Build history of the part. All positions in model axes, mm. Face numbers are marked on the shaded views. A direction names the side the tool comes from. Round coordinates to 2 decimals unless told otherwise and drop trailing zeros. Write each loop counter-clockwise with the first axis right and the second up, starting at its lowest first coordinate (ties: lowest second). Pieces come first, ordered by that corner, then holes.
1) Flat gauge pins, fed straight in: pin 1 (10 mm diameter, centred on y = 2, z = -17, fed in from +X); pin 2 (6 mm diameter, centred on x = 15, z = 27.5, fed in from -Y); pin 3 (7 mm diameter, centred on x = 0, z = 0, fed in from -Y); pin 4 (3 mm diameter, centred on x = 1.5, y = -0.5, fed in from -Z). Where does each tip first touch, or does it go through?
2) Wall check: probe 1 along Z at (x, y) = (0, 4); probe 2 along Z at (x, y) = (0, -4); probe 3 along Y at (x, z) = (10, 27.5). Give the ranges that are in metal, low to high.
3) Saw through at D-D (x = -28). Write the cut outline in (y, z).
4) Saw through at A-A (z = 1). Write the cut outline in (x, y).
5) Saw through at C-C (y = 12.5). Write the cut outline in (x, z).
6) Saw through at B-B (x = -1.5). Write the cut outline in (y, z), plus the area to 3 significant figures.
7) Which spindle directions (+Z, -Z, +X, -X, +Y, -Y) get a long thin tool onto all of the face, cutting with end or side? Do the marked faces 1 and 2. Say none if no direction does.
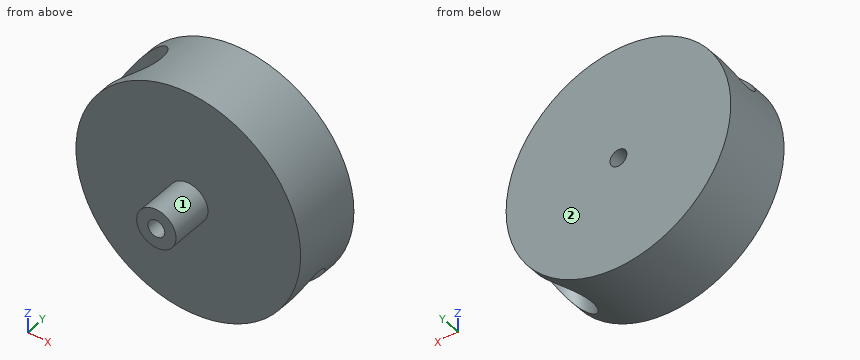
from build123d import *

# Parameters (mm, degrees)
SKETCH1_R           = 40
SKETCH1_R_2         = 3
BOSS_EXTRUDE1_DEPTH = 25
SKETCH2_R           = 7
SKETCH2_R_2         = 3
BOSS_EXTRUDE2_DEPTH = 15
SKETCH3_R           = 9
CUT_EXTRUDE1_DEPTH  = 41
SKETCH4_R           = 9
CUT_EXTRUDE2_DEPTH  = 41.0000001


with BuildPart() as part:
    # Sketch1 → Boss-Extrude1 (new body)
    with BuildSketch(Plane(origin=(0, 0, 0), x_dir=(1, 0, 0), z_dir=(0, 1, 0))):
        Circle(SKETCH1_R)
        Circle(SKETCH1_R_2, mode=Mode.SUBTRACT)
    extrude(amount=BOSS_EXTRUDE1_DEPTH)

    # Sketch2 → Boss-Extrude2 (add)
    with BuildSketch(Plane.XZ):
        Circle(SKETCH2_R)
        Circle(SKETCH2_R_2, mode=Mode.SUBTRACT)
    extrude(amount=BOSS_EXTRUDE2_DEPTH)

    # Sketch3 → Cut-Extrude1 (cut, through all)
    with BuildSketch(Plane.XY):
        with Locations((28, 12.5)):
            Circle(SKETCH3_R)
    extrude(amount=-CUT_EXTRUDE1_DEPTH, mode=Mode.SUBTRACT)

    # Sketch4 → Cut-Extrude2 (cut, through all)
    with BuildSketch(Plane.XY):
        with Locations((-28, 12.5)):
            Circle(SKETCH4_R)
    extrude(amount=CUT_EXTRUDE2_DEPTH, mode=Mode.SUBTRACT)


solid = part.part
Evaluation:
1. pin 1: stops at x = 38.16
1. pin 2: stops at y = 0
1. pin 3: stops at y = -15
1. pin 4: stops at z = -40
2. probe 1: z = -40 to -3, 3 to 40
2. probe 2: z = -7 to -3, 3 to 7
2. probe 3: y = 0 to 25
3. outline: (0, -28.57) - (25, -28.57) - (25, 28.57) - (21.5, 28.57) - (21.5, 0) - (3.5, 0) - (3.5, 28.57) - (0, 28.57) - close
4. outline: (-39.99, 0) - (-6.93, 0) - (-6.93, -15) - (-2.83, -15) - (-2.83, 25) - (-39.99, 25) - close; (2.83, -15) - (6.93, -15) - (6.93, 0) - (39.99, 0) - (39.99, 25) - (2.83, 25) - close; hole circle Ø18 at (-28, 12.5)
5. outline: (-37, 0) - (-37, 15.2) arc R40 ccw to (19, -35.2) - (19, 0) - (37, 0) - (37, -15.2) arc R40 ccw to (-19, 35.2) - (-19, 0) - close; hole circle Ø6 at (0, 0)
6. outline: (-15, -6.84) - (0, -6.84) - (0, -39.97) - (25, -39.97) - (25, -2.6) - (-15, -2.6) - close; (-15, 2.6) - (25, 2.6) - (25, 39.97) - (0, 39.97) - (0, 6.84) - (-15, 6.84) - close
6. area: 2,000 mm2
7. face 1: -Y
7. face 2: +Z, -Z, +X, -X, +Y
